from build123d import *

# Parameters (mm, degrees)
F0_R     = 120
F0_R_2   = 115
F1_DEPTH = 55
F3_DEPTH = 5
F5_DEPTH = 110.001
F6_R     = 6.35
F7_DEPTH = 254


# Not quite as in the source:
# - a pattern or mirror of a feature is missing from the dataset's text; its kind, count and spacing are read off the source's solid


with BuildPart() as f1:
    # F0 (on Front) → F1 (new body, symmetric)
    with BuildSketch(Plane.XZ):
        Circle(F0_R)
        Circle(F0_R_2, mode=Mode.SUBTRACT)
    extrude(amount=F1_DEPTH, both=True)

    # F2 (on face) → F3 (join)
    with BuildSketch(Plane(origin=(0, 55, 0), x_dir=(-1, 0, 0), z_dir=(0, 1, 0))):
        with BuildLine():
            Line((60, -103.9230484541), (75, -129.9038105677))
            ThreePointArc((75, -129.9038105677), (150, 0), (75, 129.9038105677))
            Line((75, 129.9038105677), (60, 103.9230484541))
            ThreePointArc((60, 103.9230484541), (103.9230484541, 60), (120, 0))
            ThreePointArc((120, 0), (103.9230484541, -60), (60, -103.9230484541))
        make_face()
    extrude(amount=-F3_DEPTH)

    # F4 (on face) → F5 (cut, through all)
    with BuildSketch(Plane(origin=(0, 55, 0), x_dir=(-1, 0, 0), z_dir=(0, 1, 0))):
        with BuildLine():
            ThreePointArc((134.8666666667, 5.9985183356), (134.9666625504, 3), (135, 0))
            ThreePointArc((135, 0), (134.9666625504, -3), (134.8666666667, -5.9985183356))
            ThreePointArc((134.8666666667, -5.9985183356), (139.1952353927, -4.2895221179), (141, 0))
            ThreePointArc((141, 0), (139.1952353927, 4.2895221179), (134.8666666667, 5.9985183356))
        make_face()
        with BuildLine():
            ThreePointArc((134.8666666667, -5.9985183356), (134.9666625504, -3), (135, 0))
            ThreePointArc((135, 0), (134.9666625504, 3), (134.8666666667, 5.9985183356))
            ThreePointArc((134.8666666667, 5.9985183356), (129, 0), (134.8666666667, -5.9985183356))
        make_face()
    f5 = extrude(amount=-F5_DEPTH, mode=Mode.SUBTRACT)

    # F5_copies: F5 across plane
    add(f5.mirror(Plane(origin=(0, 0, 0), x_dir=(-0.9238795325, 0, -0.3826834324), z_dir=(0.3826834324, 0, -0.9238795325))), mode=Mode.SUBTRACT)

    # F5_copies1: F5 across plane
    add(f5.mirror(Plane(origin=(0, 0, 0), x_dir=(0.9238795325, 0, -0.3826834324), z_dir=(0.3826834324, 0, 0.9238795325))), mode=Mode.SUBTRACT)

    # F6 (on Right) → F7 (cut, symmetric)
    with BuildSketch(Plane.YZ):
        Circle(F6_R)
    extrude(amount=F7_DEPTH, both=True, mode=Mode.SUBTRACT)


solid = f1.part
The listing builds one solid part. Answer for the finished solid, in the listing's coordinates (mm). A direction names the side the tool comes from. Round coordinates to 2 decimals unless told otherwise and drop trailing zeros. Order: outer loops, then holes, each group sorted by start corner. A loop starts at its lowest first (then second) coordinate and runs counter-clockwise, first axis right, second up. Notation, with made-up numbers: (50, 16) -> (88, 16) arc R11 ccw to (88, 23) -> close; hole circle Ø11 at (30.5, 9.5). An arc over 180 degrees is marked (long way). One line per item, written item: value.
Item 1: Find section C-C, the plane y = 45. Give the vertices of the cut face in (x, z).
Taken from the geometry:
outline: circle Ø240 at (0, 0); hole circle Ø230 at (0, 0)
Item 2: For a pull along Z with two mould halves and no side action, classify faces 1 (the cylindrical face through (110.85, -0.77, -45.96)), 2 (the flat face through (-67.605, 52.535, 117.095)), 3 (the cylindrical face through (106.23, 0.77, -44.05)) as released by +Z, released by -Z, zero draft, split by the parting line, or undercut.
Taken from the geometry:
face 1: split by the parting line
face 2: released by +Z
face 3: undercut
Item 3: For faces 4 (the flat face through (8, -55, -115)), 5 (the flat face through (-67.395, 52.535, -116.732)), 6 (the flat face through (-121, 50, -9)), determine the directions among +Z, -Z, +X, -X, +Y, -Y from which every point of the face is accessible in a straight line to the end or side of a thin tool.
Taken from the geometry:
face 4: +Z, -Z, +X, -X, -Y
face 5: -Z, +Y, -Y
face 6: -X, -Y
Item 4: Find section B-B, the plane z = 49. Give the vertices of the cut face in (x, y), then the cut area to 3 significant figures.
Taken from the geometry:
outline: (-141.77, 50) -> (-109.54, 50) -> (-109.54, -55) -> (-104.04, -55) -> (-104.04, 55) -> (-141.77, 55) -> close; (104.04, -55) -> (109.54, -55) -> (109.54, 55) -> (104.04, 55) -> close
area: 1,370 mm2
Item 5: Find section A-A, the plane x = 0. Give the vertices of the cut face in (y, z), then the cut area to 3 significant figures.
Taken from the geometry:
outline: (-55, -120) -> (55, -120) -> (55, -115) -> (-55, -115) -> close; (-55, 115) -> (55, 115) -> (55, 120) -> (-55, 120) -> close
area: 1,100 mm2
Item 6: Given P1, Ø7.5, axis at y = 0, z = 0, coming from the -X side; P2, Ø1, axis at x = -105.5, z = 81.5, coming from the -Y side; P3, Ø8, axis at y = -23.5, z = -62.5, coming from the +X side; P4, Ø6, axis at x = -67, y = -39.5, coming from the +Z side, each flat-ended and moving along its own axis, determine where each tip first touches the part or whether it passes through.
Taken from the geometry:
P1: passes through
P2: stops at y = 50
P3: stops at x = 104.77
P4: stops at z = 101.51
Item 7: Straight lines are drawn through the part: L1, parallel to Z at x = 0, y = 27; L2, parallel to Y at x = 116.1, z = 0; L3, parallel to Z at x = 21.5, y = -2. For each, find the intervals that lie inside material, in ascending order.
Taken from the geometry:
L1: z = -120 to -115, 115 to 120
L2: y = -55 to -6.35, 6.35 to 55
L3: z = -118.06 to -112.97, 112.97 to 118.06
